The listing builds one solid part. Answer for the finished solid, in the listing's coordinates (mm). A direction names the side the tool comes from. Round coordinates to 2 decimals unless told otherwise and drop trailing zeros. Loops run counter-clockwise (first coordinate to the right, second up) from the corner with the lowest first, then second, coordinate; pieces in that order, holes last. Notation, with made-up numbers: (-38.5, 66) - (10.5, 66) arc R21 cw to (10.5, 78) - close; hole circle Ø1 at (-35, 83.25). An arc over 180 degrees is marked (long way). Write item = value, one per line. Start each with the question number.
1) Section C-C, the plane y = 7.5 is taken. Determine the outline of the cut face in (x, z), and give its area (4 significant figures).
2) Section B-B, the plane z = 10.75 is taken. Determine the outline of the cut face in (x, y), and give its area (3 significant figures).
3) A tool of negligible diameter and unlimited length cuts with its end or side. For faces 1 (the cylindrical face through (-11.77, -1.48, 7.6)), 2 (the flat face through (0, 5, 7)), 3 (the flat face through (32.6, -5.1, 7.4)), from which of +Z, -Z, +X, -X, +Y, -Y can it reach the whole face along a straight path? Write none if from no direction.
4) For a pull along X with two mould halves and no side action, classify faces 4 (the flat face through (0, 1, 0)), 5 (the cylindrical face through (11.77, -1.48, 7.6)), 6 (the cylindrical face through (-12.58, 12.34, 7.39)) as released by +X, released by -X, zero draft, split by the parting line, or undercut.
5) Straight lines are drawn through the part: line 1 along X through (y, z) = (9, 2.5); line 2 along X through (y, z) = (-12.5, 5.25); line 3 along X through (y, z) = (3, 10.25). For each, find the intervals that lie inside material, in ascending order.
6) Section A-A, the plane y = -9 is taken. Determine the outline of the cut face in (x, z), and give its area (3 significant figures).
7) Given pin 1 Ø6 at (x, y) = (18.5, 1) entering from -Z; pin 2 Ø1 at (x, z) = (2, 3.5) entering from +Y; pin 3 Ø8 at (x, z) = (24.5, 5.5) entering from +Y; pin 4 Ø5 at (y, z) = (10.5, 10.5) entering from +X, each flat-ended and moving along its own axis, determine where each tip first touches the part or whether it passes through.
8) Section D-D, the plane x = -1 is taken. Determine the outline of the cut face in (y, z), and give its area (3 significant figures).
from build123d import *

# Parameters (mm, degrees)
ESTRUSIONE_ESTRUSIONE1_DEPTH = 15
RACCORDO1_R                  = 30
RACCORDO2_R                  = 20


with BuildPart() as part:
    # Schizzo2 → Estrusione-Estrusione1 (new body)
    with BuildSketch(Plane.XY):
        with BuildLine():
            Line((12.5, 0), (-12.5, 0))
            Line((-12.5, 0), (-37.248737342, -24.748737342))
            ThreePointArc((-37.248737342, -24.748737342), (-42.410299766, -22.234372931), (-44.319805153, -16.819805153))
            Line((-44.319805153, -16.819805153), (-12.5, 15))
            Line((-12.5, 15), (-2.75, 15))
            Line((-2.75, 15), (-2.75, 5))
            Line((-2.75, 5), (2.75, 5))
            Line((2.75, 5), (2.75, 15))
            Line((2.75, 15), (12.5, 15))
            Line((12.5, 15), (44.319805153, -16.819805153))
            ThreePointArc((44.319805153, -16.819805153), (42.410299766, -22.234372931), (37.248737342, -24.748737342))
            Line((37.248737342, -24.748737342), (12.5, 0))
        make_face()
    extrude(amount=ESTRUSIONE_ESTRUSIONE1_DEPTH)

    # Raccordo1
    # the kernel refuses this fillet: 30 mm, written as the material it takes off along each edge
    with BuildSketch(Plane(origin=(12.5, 15, -30.600334507), x_dir=(-1, 0, 0), z_dir=(0, 0, 1))) as raccordo1_piece_1:
        with BuildLine():
            CenterArc((12.558121821, 29.86828505), RACCORDO1_R, 225, 39.629019647)
            Line((-8.655081615, 8.655081615), (-9.079345683, 8.230817546))
            Line((-9.079345683, 8.230817546), (-0.424264069, -0.424264069))
            Line((-0.424264069, -0.424264069), (0, -0.6))
            ThreePointArc((0, -0.6), (4.875, -0.6), (9.693837564, -0.597365701))
            Line((9.693837564, -0.597365701), (9.75, 0))
        make_face()
    extrude(amount=76.200669014, mode=Mode.SUBTRACT)
    with BuildSketch(Plane(origin=(-12.5, 15, -30.600334507), x_dir=(-0.7071067811865485, -0.7071067811865467, 0), z_dir=(0, 0, 1))) as raccordo1_piece_2:
        with BuildLine():
            CenterArc((12.240133803, 30), RACCORDO1_R, 230.370980353, 39.629019647)
            Line((-6.894291117, 6.894291117), (-7.276979615, 6.432176939))
            ThreePointArc((-7.276979615, 6.432176939), (-3.871409627, 3.02288149), (-0.424264069, -0.424264069))
            Line((-0.424264069, -0.424264069), (0, -0.6))
            Line((0, -0.6), (12.240133803, -0.6))
            Line((12.240133803, -0.6), (12.240133803, 0))
        make_face()
    extrude(amount=76.200669014, mode=Mode.SUBTRACT)

    # Raccordo2
    raccordo2_edges = [part.edges().sort_by_distance(p)[0] for p in [
        (12.5, 0, 7.5),
        (-12.5, 0, 7.5),
    ]]
    fillet(raccordo2_edges, radius=RACCORDO2_R)


solid = part.part
Geometry check:
q1.outline = (-19.93, 0) - (-2.75, 0) - (-2.75, 15) - (-19.93, 15) - close; (2.75, 0) - (19.93, 0) - (19.93, 15) - (2.75, 15) - close
q1.area = 515.5 mm2
q2.outline = (-44.32, -16.82) arc R7.56 ccw to (-37.25, -24.75) - (-18.36, -5.86) arc R20 cw to (-4.22, 0) - (4.22, 0) arc R20 cw to (18.36, -5.86) - (37.25, -24.75) arc R7.56 ccw to (44.32, -16.82) - (21.16, 6.34) arc R30 ccw to (2.75, 15) - (2.75, 5) - (-2.75, 5) - (-2.75, 15) arc R30 ccw to (-21.16, 6.34) - close
q2.area = 1,180 mm2
q3.face_1 = +Z, -Z, -Y
q3.face_2 = +Z, -Z, +Y
q3.face_3 = +Z, -Z, +X, +Y
q4.face_4 = zero draft
q4.face_5 = undercut
q4.face_6 = released by -X
q5.line_1 = -18.12 to -2.75, 2.75 to 18.12
q5.line_2 = -40 to -25, 25 to 40
q5.line_3 = -24.5 to 24.5
q6.outline = (-36.5, 0) - (-21.5, 0) - (-21.5, 15) - (-36.5, 15) - close; (21.5, 0) - (36.5, 0) - (36.5, 15) - (21.5, 15) - close
q6.area = 450 mm2
q7.pin_1 = 0
q7.pin_2 = 5
q7.pin_3 = 6.98
q7.pin_4 = 19.36
q8.outline = (0, 0) - (5, 0) - (5, 15) - (0, 15) - close
q8.area = 75.0 mm2
